Source: CAD feature listing. Evaluate the final solid. Frame: model axes, mm. Coordinates: 2 decimals unless noted, no trailing zeros. Order: outer loops, then holes, each group sorted by start corner. A loop starts at its lowest first (then second) coordinate and runs counter-clockwise, first axis right, second up. Notation, with made-up numbers: (40, 3) -> (83, 3) arc R29 ccw to (83, 30) -> close; hole circle Ø1 at (86, 42.25). An arc over 180 degrees is marked (long way). Write item = value, one per line. Start each with the question number.
Item 1: Contact query for flat-ended pins moving along their axis: pin 1 (2 mm diameter, centred on x = 54, z = 10.5, fed in from +Y); pin 2 (10 mm diameter, centred on x = 35, z = 12.5, fed in from +Y). Output: stop coordinate, or through.
Item 2: Ray query, line 1 along Y through (x, z) = (62, 29); line 2 along X through (y, z) = (21.5, 26); line 3 along Y through (x, z) = (43.5, 2). Return the intervals inside material, ascending. Write a range as [from, to].
Item 3: Section query B-B (y = 44). Output: boundary loops of the cut face in (x, z).
Item 4: Section query A-A (x = 47). Output: boundary loops of the cut face in (y, z).
```python
from build123d import *

# Parameters (mm, degrees)
EXTRUDE_1_DEPTH = 35


with BuildPart() as part:
    # 草圖2 → 填料-伸長1 (new body)
    with BuildSketch(Plane.XY):
        with BuildLine():
            Line((0, 0), (0, 50))
            Line((0, 50), (28, 50))
            Line((28, 50), (51.956313103, 42.44328469))
            add(Edge.make_bspline(
                [(51.956313103, 42.44328469), (83.897076516, 4.556034867), (124.627264654, 70.257246507), (150, 19.209377101)],
                knots=[0, 0, 0, 0, 1, 1, 1, 1], degree=3))
            Line((150, 19.209377101), (150, 0))
            Line((150, 0), (0, 0))
        make_face()
    extrude(amount=EXTRUDE_1_DEPTH)


solid = part.part
```
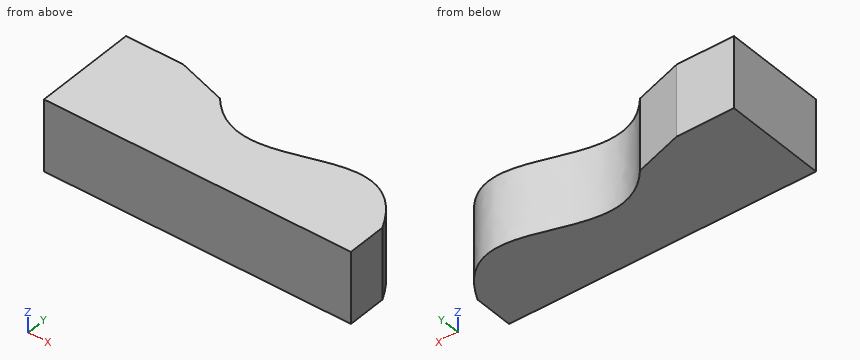
Computed:
q1.pin_1 = 41.25
q1.pin_2 = 49.37
q2.line_1 = [0, 33.84]
q2.line_2 = [0, 148.81]
q2.line_3 = [0, 45.11]
q3.outline = (0, 0) -> (47.02, 0) -> (47.02, 35) -> (0, 35) -> close
q4.outline = (0, 0) -> (44.01, 0) -> (44.01, 35) -> (0, 35) -> close
